```python
from build123d import *

# Parameters (mm, degrees)
SKETCH1_W          = 177.8
SKETCH1_H          = 19.812
BASE_DEPTH         = 4.826
SKETCH2_W          = 34.925
SKETCH2_H          = 4.826
SKETCH2_W_2        = 19.05
TOP_TABS_DEPTH     = 179.965487231
SKETCH3_W          = 60.325
SKETCH3_H          = 4.826
SKETCH3_W_2        = 19.05
CUT_EXTRUDE2_DEPTH = 179.965487231


with BuildPart() as part:
    # Sketch1 → Base (new body)
    with BuildSketch(Plane(origin=(0, 0, 0), x_dir=(0, 0, -1), z_dir=(1, 0, 0))):
        with Locations((88.9, 9.906)):
            Rectangle(SKETCH1_W, SKETCH1_H)
    extrude(amount=BASE_DEPTH)

    # Sketch2 → Top Tabs (cut, through all)
    with BuildSketch(Plane(origin=(4.826, 0, 0), x_dir=(0, 0, -1), z_dir=(1, 0, 0))):
        with Locations((68.2625, 17.399)):
            Rectangle(SKETCH2_W, SKETCH2_H)
        with Locations((114.3, 17.399)):
            Rectangle(SKETCH2_W_2, SKETCH2_H)
        with Locations((160.3375, 17.399)):
            Rectangle(SKETCH2_W, SKETCH2_H)
    extrude(amount=-TOP_TABS_DEPTH, mode=Mode.SUBTRACT)

    # Sketch3 → Cut-Extrude2 (cut, through all)
    with BuildSketch(Plane(origin=(4.826, 0, 0), x_dir=(0, 0, -1), z_dir=(1, 0, 0))):
        with Locations((30.1625, 2.413)):
            Rectangle(SKETCH3_W, SKETCH3_H)
        with Locations((147.6375, 2.413)):
            Rectangle(SKETCH3_W, SKETCH3_H)
        with Locations((88.9, 2.413)):
            Rectangle(SKETCH3_W_2, SKETCH3_H)
    extrude(amount=-CUT_EXTRUDE2_DEPTH, mode=Mode.SUBTRACT)


solid = part.part
```
Read the model definition and answer for the solid it produces. Units are mm, in the model's axes. A direction names the side the tool comes from. Give positions to 0.01 mm unless a question says otherwise; leave off trailing zeros. Write each loop counter-clockwise with the first axis right and the second up, starting at its lowest first coordinate (ties: lowest second). Pieces come first, ordered by that corner, then holes. Notation, with made-up numbers: (-38, 13.5) -> (-5, 13.5) arc R20 ccw to (-5, 50.5) -> close; hole circle Ø2 at (-39.5, 39). An arc over 180 degrees is marked (long way). Answer as a JSON object with one key per item and string values.
1) Section A-A on x = 1.2 is taken. Write down the section's boundary in (y, z) (3 decimals), then the cut area to 3 significant figures.
Findings below:
{"outline": "(0, -117.475) -> (4.826, -117.475) -> (4.826, -177.8) -> (14.986, -177.8) -> (14.986, -142.875) -> (19.812, -142.875) -> (19.812, -123.825) -> (14.986, -123.825) -> (14.986, -104.775) -> (19.812, -104.775) -> (19.812, -85.725) -> (14.986, -85.725) -> (14.986, -50.8) -> (19.812, -50.8) -> (19.812, 0) -> (4.826, 0) -> (4.826, -60.325) -> (0, -60.325) -> (0, -79.375) -> (4.826, -79.375) -> (4.826, -98.425) -> (0, -98.425) -> close", "area": "2,420 mm^2"}
2) Straight lines are drawn through the part: probe 1 along Z at (x, y) = (3.3, 17.25) (3 decimals); probe 2 along Z at (x, y) = (1.45, 4.25) (3 decimals); probe 3 along Y at (x, z) = (0.7, -98). For each, find the intervals that lie inside material, in ascending order. Write a range as from..to.
Findings below:
{"probe 1": "z = -142.875..-123.825, -104.775..-85.725, -50.8..0", "probe 2": "z = -117.475..-98.425, -79.375..-60.325", "probe 3": "y = 4.83..19.81"}
3) A tool of negligible diameter and unlimited length cuts with its end or side. For faces 4 (the flat face through (2, 17, -123.825)), 5 (the flat face through (2, 2, -117.475)), 6 (the flat face through (2, 2, -98.425)), from which of +Z, -Z, +X, -X, +Y, -Y can it reach the whole face along a straight path? Write none if from no direction.
Findings below:
{"face 4": "+X, -X, +Y", "face 5": "-Z, +X, -X, -Y", "face 6": "+X, -X, -Y"}
4) Section B-B on z = -91 is taken. Write down the section's boundary in (x, y), then the cut area to 3 significant figures.
Findings below:
{"outline": "(0, 4.83) -> (4.83, 4.83) -> (4.83, 19.81) -> (0, 19.81) -> close", "area": "72.3 mm^2"}
5) For a pull along Z with two mould halves and no side action, classify faces 1 (the flat face through (2, 4.826, -147)), 2 (the flat face through (2, 2, -60.325)), 3 (the flat face through (2, 14.986, -114)) as pulls with the +Z half, pulls with the -Z half, needs draft (parallel to the pull), parting line crosses it, or undercut.
Findings below:
{"face 1": "needs draft", "face 2": "pulls with the +Z half", "face 3": "undercut"}
6) Flat-ended cylindrical pins translate along their axes: pin 1 Ø2.5 at (x, y) = (2.5, 2) entering from -Z (3 decimals); pin 2 Ø2.5 at (x, z) = (2, -34.5) entering from -Y; pin 3 Ø1.4 at (x, z) = (1.5, -162) entering from +Y. Find the tip coordinate at first contact, or state that the pin passes through.
Findings below:
{"pin 1": "stops at z = -117.475", "pin 2": "stops at y = 4.83", "pin 3": "stops at y = 14.99"}
